Source: CAD feature listing. Evaluate the final solid. Frame: model axes, mm. A direction names the side the tool comes from. Give positions to 0.01 mm unless a question says otherwise; leave off trailing zeros. Put each result on its own line as item: value.
```python
from build123d import *

# Parameters (mm, degrees)
SKETCH1_W           = 33
SKETCH1_H           = 28
BOSS_EXTRUDE1_DEPTH = 46
CUT_EXTRUDE1_DEPTH  = 59.318093247
CUT_EXTRUDE2_START  = -3
CUT_EXTRUDE2_DEPTH  = 27
FILLET1_R           = 12.5
FILLET2_R           = 16.5
FILLET3_R           = 6
SKETCH4_W           = 13
SKETCH4_H           = 23
CUT_EXTRUDE3_DEPTH  = 9
SKETCH5_R           = 6.5
CUT_EXTRUDE4_DEPTH  = 56.592265809
SKETCH6_R           = 1
CUT_EXTRUDE5_DEPTH  = 8
SKETCH7_R           = 1.3
SKETCH7_R_2         = 2.5
CUT_EXTRUDE6_DEPTH  = 2.5


with BuildPart() as part:
    # Sketch1 → Boss-Extrude1 (new body)
    with BuildSketch(Plane.XY):
        Rectangle(SKETCH1_W, SKETCH1_H)
    extrude(amount=BOSS_EXTRUDE1_DEPTH)

    # Sketch2 → Cut-Extrude1 (cut, through all)
    with BuildSketch(Plane(origin=(16.5, 0, 0), x_dir=(0, 0, -1), z_dir=(1, 0, 0))):
        with BuildLine():
            Line((-5, -14), (-46, -14))
            Line((-46, -14), (-46, 2))
            add(Edge.make_bspline(
                [(-46, 2), (-24.29854511, -1.646485385), (-5, -14)],
                knots=[0, 0, 0, 1, 1, 1], degree=2))
        make_face()
    extrude(amount=-CUT_EXTRUDE1_DEPTH, mode=Mode.SUBTRACT)

    # Sketch3 → Cut-Extrude2 (cut)
    with BuildSketch(Plane(origin=(16.5, 0, 0), x_dir=(0, 0, -1), z_dir=(1, 0, 0)).offset(CUT_EXTRUDE2_START)):
        with BuildLine():
            Line((-5, -14), (-2.5, -14))
            Line((-2.5, -14), (-2.5, 3.5))
            Line((-2.5, 3.5), (-40.5, 3.5))
            Line((-40.5, 3.5), (-40.5, 0.927448298))
            add(Edge.make_bspline(
                [(-5, -14), (-21.835639292, -3.223057237), (-40.5, 0.927448298)],
                knots=[0, 0, 0, 1, 1, 1], degree=2))
        make_face()
    extrude(amount=-CUT_EXTRUDE2_DEPTH, mode=Mode.SUBTRACT)

    # Fillet1
    fillet1_edges = [part.edges().sort_by_distance(p)[0] for p in [
        (13.5, 2.213724149, 40.5),
        (-13.5, 2.213724149, 40.5),
    ]]
    fillet(fillet1_edges, radius=FILLET1_R)

    # Fillet2
    fillet2_edges = [part.edges().sort_by_distance(p)[0] for p in [
        (16.5, 8, 46),
        (-16.5, 8, 46),
    ]]
    fillet(fillet2_edges, radius=FILLET2_R - 0.0001)  # a hair under: the kernel refuses the full size

    # Fillet3
    fillet3_edges = [part.edges().sort_by_distance(p)[0] for p in [
        (16.5, -14, 2.5),
        (-16.5, -14, 2.5),
    ]]
    fillet(fillet3_edges, radius=FILLET3_R)

    # Sketch4 → Cut-Extrude3 (cut)
    with BuildSketch(Plane.XZ.offset(-3.5)):
        with Locations((0, 20.5)):
            Rectangle(SKETCH4_W, SKETCH4_H)
    extrude(amount=-CUT_EXTRUDE3_DEPTH, mode=Mode.SUBTRACT)

    # Sketch5 → Cut-Extrude4 (cut, through all)
    with BuildSketch(Plane.XZ.offset(-12.5)):
        with Locations(Location((0, 25.5, 0), (0, 0, 270))):
            Circle(SKETCH5_R)
    extrude(amount=-CUT_EXTRUDE4_DEPTH, mode=Mode.SUBTRACT)

    # Sketch6 → Cut-Extrude5 (cut)
    with BuildSketch(Plane.XZ.offset(-3.5)):
        with Locations(Location((0, 34.034163798, 0), (0, 0, 270))):
            Circle(SKETCH6_R)
        with Locations(Location((0, 6.434163798, 0), (0, 0, 270))):
            Circle(SKETCH6_R)
    extrude(amount=-CUT_EXTRUDE5_DEPTH, mode=Mode.SUBTRACT)

    # Sketch7 → Cut-Extrude6 (cut)
    with BuildSketch(Plane(origin=(0, 0, 0), x_dir=(-1, 0, 0), z_dir=(0, 0, -1))):
        with Locations((-0.5, 0)):
            Circle(SKETCH7_R)
        with Locations((-5, 0)):
            Circle(SKETCH7_R_2)
        with Locations((-9.5, 0)):
            Circle(SKETCH7_R)
    extrude(amount=-CUT_EXTRUDE6_DEPTH, mode=Mode.SUBTRACT)


solid = part.part
```
(1) First-contact query: P1, Ø5, axis at x = -5.5, y = -8.5, coming from the +Z side; P2, Ø0.6, axis at x = 0, z = 34, coming from the -Y side; P3, Ø3, axis at x = -9, z = 34.5, coming from the -Y side. Flat tips, straight axial feed; report the tip coordinate or a pass-through.
Calculated:
P1: stops at z = 2.5
P2: stops at y = 11.5
P3: stops at y = 3.5
(2) Section A-A on y = 6.5. Give the number of separate pieces and of enclosed holes in the cut face, then the cut area to 3 significant figures.
Calculated:
separate pieces: 1
enclosed holes: 3
area: 1,100 mm²
(3) Line query: probe 1 along Y at (x, z) = (5, 1); probe 2 along X at (y, z) = (-7.25, 12.5); probe 3 along X at (y, z) = (10.75, 29). Output: solid intervals per line, ascending. Write a range as from..to.
Calculated:
probe 1: y = -14..-2.5, 2.5..14
probe 2: x = -16.5..-13.5, 13.5..16.5
probe 3: x = -16.5..-6.5, 6.5..16.5
(4) Draft query along Z for faces 4 (the flat face through (-6.5, 8, 20)), 5 (the cylindrical face through (2.615, 0.751, 1.232)), 6 (the cylindrical face through (11.795, 7.833, 41.038)). Return one class per face: released by +Z, released by -Z, zero draft, split by the parting line, or undercut.
Calculated:
face 4: undercut
face 5: zero draft
face 6: released by +Z
(5) Reachability of faces 1 (the flat face through (5, 12.5, 31)), 2 (the cylindrical face through (15.965, -10.476, 4.421)), 3 (the cylindrical face through (8.26, 0.39, 1.23)) from +Z, -Z, +X, -X, +Y, -Y: full face, straight path, thin tool, end or side. Return the list, or none.
Calculated:
face 1: -Y
face 2: +Z, -Z, +X, -Y
face 3: -Z
